from build123d import *

# Parameters (mm, degrees)
F0_W     = 73.66
F0_H     = 36.738612
F1_DEPTH = 10.922
F2_R     = 5.08


with BuildPart() as f1:
    # F0 (on Top) → F1 (new body, symmetric)
    with BuildSketch(Plane.XY):
        Rectangle(F0_W, F0_H)
    extrude(amount=F1_DEPTH, both=True)

    # F2
    f2_edges = [f1.edges().sort_by_distance(p)[0] for p in [
        (-36.83, 0, 10.922),
        (0, -18.369306, 10.922),
        (0, 18.369306, 10.922),
    ]]
    fillet(f2_edges, radius=F2_R)


solid = f1.part
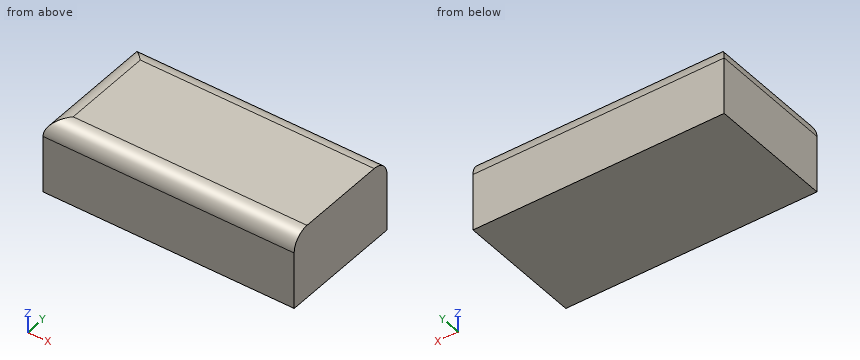
The listing builds one solid part. Answer for the finished solid, in the listing's coordinates (mm). Give positions to 0.01 mm unless a question says otherwise; leave off trailing zeros. Order: outer loops, then holes, each group sorted by start corner. A loop starts at its lowest first (then second) coordinate and runs counter-clockwise, first axis right, second up. Notation, with made-up numbers: (65, 39) - (70, 39) arc R20 cw to (70, 76) - close; hole circle Ø9 at (10, 41.5). An arc over 180 degrees is marked (long way). One line per item, written item: value. Start each with the question number.
1) A cutting plane is placed at A-A on y = 16. Give the vertices of the cut face in (x, z).
2) Given pin 1 Ø1 at (x, y) = (9, 14) entering from +Z, flat-ended and moving along its own axis, determine where the tip first touches the part or whether it passes through.
3) Find the intervals of material crossed by L1, parallel to Y at x = -33, z = 6; L2, parallel to Z at x = -34, y = -12; L3, parallel to Z at x = 0.5, y = 16.5, in increasing order.
Answer sheet:
1. outline: (-36.83, -10.92) - (36.83, -10.92) - (36.83, 10.14) - (-34.46, 10.14) arc R5.08 ccw to (-36.83, 5.84) - close
2. pin 1: stops at z = 10.92
3. L1: y = -18.37 to 18.37
3. L2: z = -10.92 to 10.4
3. L3: z = -10.92 to 9.78
